For this review, take the finished solid that the model builds, in its own axes (mm). A direction names the side the tool comes from. Round coordinates to 2 decimals unless told otherwise and drop trailing zeros. Loops run counter-clockwise (first coordinate to the right, second up) from the corner with the lowest first, then second, coordinate; pieces in that order, holes last.
```python
from build123d import *

# Parameters (mm, degrees)
F0_R     = 11
F1_DEPTH = 6.2
F2_R     = 5
F3_DEPTH = 6.5
F4_R     = 2
F5_DEPTH = 25


with BuildPart() as f1:
    # F0 (on Front) → F1 (new body)
    with BuildSketch(Plane.XZ):
        Circle(F0_R)
    extrude(amount=F1_DEPTH)

    # F2 (on face) → F3 (join)
    with BuildSketch(Plane(origin=(0, 0, 0), x_dir=(-1, 0, 0), z_dir=(0, 1, 0))):
        Circle(F2_R)
    extrude(amount=F3_DEPTH)

    # F4 (on face) → F5 (cut)
    with BuildSketch(Plane(origin=(0, 6.5, 0), x_dir=(-1, 0, 0), z_dir=(0, 1, 0))):
        Circle(F4_R)
    extrude(amount=-F5_DEPTH, mode=Mode.SUBTRACT)


solid = f1.part
```
(1) Add section A-A (z = 0). Give the boundary of the cut face in (x, y).
(2) For faces 1 (the cylindrical face through (1.08, 3.2, -4.88)), 2 (the cylindrical face through (-2.38, -3.06, -10.74)), list the 3-axis set-ups (+Z, -Z, +X, -X, +Y, -Y) from which the entire face can be reached by the end or side of a thin tool; tool diameter is ignored.
(3) Add section C-C (y = 0.5). Give the boundary of the cut face in (x, z), plus the area to 3 significant figures.
(4) Add section D-D (x = -2.5). Give the boundary of the cut face in (y, z).
(5) Insertion check: pin 1 Ø6 at (x, z) = (-4, 7) entering from +Y; pin 2 Ø4 at (y, z) = (3.5, 8.5) entering from +X; pin 3 Ø4 at (x, y) = (3, -3) entering from +Z. Each pin has a flat end and moves straight along its axis. Give the tip position at first contact, or say it passes through.
(6) For L1, parallel to Z at x = 0, y = -1.5; L2, parallel to Z at x = 0, y = 1.75; L3, parallel to Y at x = 8.5, z = -5, list the stretches that pass through material, from the lowest coordinate up.
(7) Add section B-B (x = 0). Give the boundary of the cut face in (y, z), plus the area to 3 significant figures.
Outcome:
1. outline: (-11, -6.2) - (-2, -6.2) - (-2, 6.5) - (-5, 6.5) - (-5, 0) - (-11, 0) - close; (2, -6.2) - (11, -6.2) - (11, 0) - (5, 0) - (5, 6.5) - (2, 6.5) - close
2. face 1: +Y
2. face 2: +Y, -Y
3. outline: circle Ø10 at (0, 0); hole circle Ø4 at (0, 0)
3. area: 66.0 mm2
4. outline: (-6.2, -10.71) - (0, -10.71) - (0, -4.33) - (6.5, -4.33) - (6.5, 4.33) - (0, 4.33) - (0, 10.71) - (-6.2, 10.71) - close
5. pin 1: stops at y = 0
5. pin 2: passes through
5. pin 3: stops at z = 10.95
6. L1: z = -11 to -2, 2 to 11
6. L2: z = -5 to -2, 2 to 5
6. L3: y = -6.2 to 0
7. outline: (-6.2, -11) - (0, -11) - (0, -5) - (6.5, -5) - (6.5, -2) - (-6.2, -2) - close; (-6.2, 2) - (6.5, 2) - (6.5, 5) - (0, 5) - (0, 11) - (-6.2, 11) - close
7. area: 151 mm2
